Verification items for the finished model (mm, model axes). Coordinates: 2 decimals unless noted, no trailing zeros. Order: outer loops, then holes, each group sorted by start corner. A loop starts at its lowest first (then second) coordinate and runs counter-clockwise, first axis right, second up. Notation, with made-up numbers: (-21.75, -32.5) -> (37.25, -32.5) arc R21 cw to (37.25, -3.5) -> close; hole circle Ø8 at (4, -32). An arc over 180 degrees is marked (long way). Write item = value, one per line. Start each with the question number.
1. Cross-section at B-B on y = -37.5. Record the cut outline in (x, z).
2. Thickness scan on line 1 along Y through (x, z) = (10, -0.6); line 2 along X through (y, z) = (-37.5, -0.3); line 3 along Y through (x, z) = (10.5, -0.6). Record the ranges inside material, lowest first. Write a range as from..to.
3. Go/stop test with a flat-tipped pin: P1, Ø8, axis at x = 4, y = 5.5, coming from the +Z side. Record where the tip stops, or that it passes through.
4. Cross-section at A-A on x = 10. Record the cut outline in (y, z).
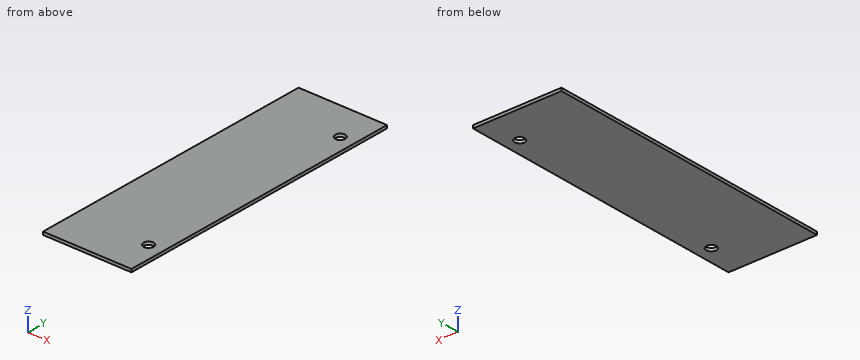
from build123d import *

# Parameters (mm, degrees)
SKETCH1_W               = 30
SKETCH1_H               = 100
BOSS_EXTRUDE1_DEPTH     = 1
CUT_EXTRUDE1_DEPTH      = 53.211109929
CUT_EXTRUDE1_DEPTH_BACK = 53.211109929
SKETCH2_R               = 1.7


with BuildPart() as part:
    # Sketch1 → Boss-Extrude1 (new body)
    with BuildSketch(Plane.XY):
        Rectangle(SKETCH1_W, SKETCH1_H)
    extrude(amount=-BOSS_EXTRUDE1_DEPTH)

    # Sketch2 → Cut-Extrude1 (cut, two sides: drawn at the far end of the back side and taken through both)
    with BuildSketch(Plane.XY.offset(-CUT_EXTRUDE1_DEPTH_BACK)):
        with Locations((10, -37.5)):
            Circle(SKETCH2_R)
        with Locations((10, 37.5)):
            Circle(SKETCH2_R)
    extrude(amount=CUT_EXTRUDE1_DEPTH + CUT_EXTRUDE1_DEPTH_BACK, mode=Mode.SUBTRACT)


solid = part.part
Worked out:
q1.outline = (-15, -1) -> (8.3, -1) -> (8.3, 0) -> (-15, 0) -> close; (11.7, -1) -> (15, -1) -> (15, 0) -> (11.7, 0) -> close
q2.line_1 = -50..-39.2, -35.8..35.8, 39.2..50
q2.line_2 = -15..8.3, 11.7..15
q2.line_3 = -50..-39.12, -35.88..35.88, 39.12..50
q3.P1 = 0
q4.outline = (-50, -1) -> (-39.2, -1) -> (-39.2, 0) -> (-50, 0) -> close; (-35.8, -1) -> (35.8, -1) -> (35.8, 0) -> (-35.8, 0) -> close; (39.2, -1) -> (50, -1) -> (50, 0) -> (39.2, 0) -> close
